Read the model definition and answer for the solid it produces. Units are mm, in the model's axes. Coordinates: 2 decimals unless noted, no trailing zeros. Order: outer loops, then holes, each group sorted by start corner. A loop starts at its lowest first (then second) coordinate and runs counter-clockwise, first axis right, second up. Notation, with made-up numbers: (88, -37.75) -> (121, -37.75) arc R20 ccw to (121, -27.75) -> close; hole circle Ø9 at (16.5, 38.25). An arc over 180 degrees is marked (long way). Answer in a Markdown table with one row per item.
from build123d import *

# Parameters (mm, degrees)
BOSS_EXTRUDE1_DEPTH = 1.5875
CUT_EXTRUDE1_DEPTH  = 4.175


with BuildPart() as part:
    # Sketch1 → Boss-Extrude1 (new body, symmetric)
    with BuildSketch(Plane.XY):
        Polygon((76.2, 37.697541537), (76.2, 56.747541537), (79.375, 56.747541537), (79.375, 37.697541537), (92.075, 37.697541537), (92.075, 46.587541537), (95.25, 46.587541537), (95.25, 37.697541537), (136.525, 37.697541537), (136.525, 46.587541537), (139.7, 46.587541537), (139.7, 37.697541537), (152.4, 37.697541537), (152.4, 69.447541537), (0, 69.447541537), (-0.423998633, 69.491926731), (-3.587863461, 69.757603883), (-946.051908629, 122.953392794), (-946.583462345, 116.623288424), (-943.412318182, 116.444298555), (-943.91275138, 110.48479854), (-6.775989292, 31.791225946), (-5.713280681, 44.446685258), (-2.549415853, 44.181008106), (-3.612124464, 31.525548794), (-1.492292584, 31.347541537), (0, 31.347541537), (0, 44.047541537), (3.175, 44.047541537), (3.175, 31.347541537), (15.875, 31.347541537), (15.875, 36.427541537), (19.05, 36.427541537), (19.05, 31.347541537), (25.4, 31.347541537), (69.85, 37.697541537), align=None)
    extrude(amount=BOSS_EXTRUDE1_DEPTH, both=True)

    # Sketch2 → Cut-Extrude1 (cut, through all)
    with BuildSketch(Plane.XY.offset(1.5875)):
        Polygon((-76.254460917, 37.625496217), (-75.245037036, 49.646404609), (-78.411328309, 49.883186), (-79.418325745, 37.891173369), align=None)
        Polygon((-155.224527027, 44.256797945), (-154.27566721, 55.556468134), (-157.441958483, 55.793249525), (-158.388391855, 44.522475098), align=None)
        Polygon((-234.194593137, 50.888099674), (-233.306297384, 61.466531659), (-236.472588657, 61.70331305), (-237.358457965, 51.153776826), align=None)
        Polygon((-313.164659247, 57.519401402), (-312.336927558, 67.376595183), (-315.503218831, 67.613376574), (-316.328524075, 57.785078555), align=None)
        Polygon((-392.134725356, 64.15070313), (-391.367557732, 73.286658708), (-394.533849005, 73.523440099), (-395.298590185, 64.416380283), align=None)
        Polygon((-471.104791466, 70.782004859), (-470.398187906, 79.196722233), (-473.564479179, 79.433503624), (-474.268656294, 71.047682011), align=None)
        Polygon((-550.074857576, 77.413306587), (-549.42881808, 85.106785757), (-552.595109353, 85.343567149), (-553.238722404, 77.67898374), align=None)
        Polygon((-629.044923686, 84.044608316), (-628.459448254, 91.016849282), (-631.625739527, 91.253630673), (-632.208788514, 84.310285468), align=None)
        Polygon((-708.014989796, 90.675910044), (-707.490078428, 96.926912807), (-710.656369701, 97.163694198), (-711.178854624, 90.941587197), align=None)
        Polygon((-786.985055905, 97.307211772), (-786.520708602, 102.836976331), (-789.686999875, 103.073757723), (-790.148920734, 97.572888925), align=None)
        Polygon((-865.955122015, 103.938513501), (-865.551338776, 108.747039856), (-868.717630049, 108.983821247), (-869.118986843, 104.204190653), align=None)
    extrude(amount=-CUT_EXTRUDE1_DEPTH, mode=Mode.SUBTRACT)


solid = part.part
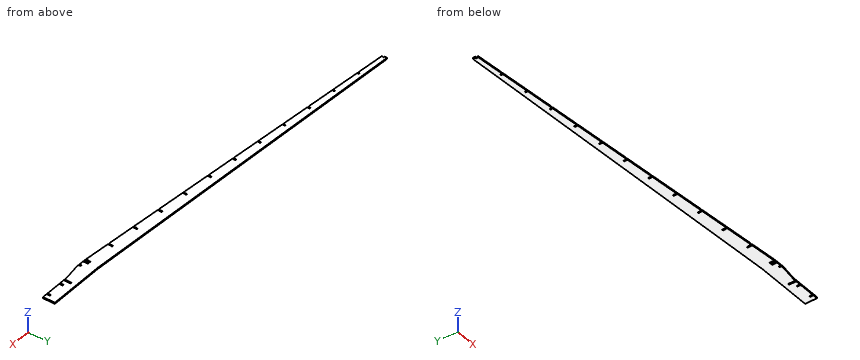
Q1. The part is cut by section B-B (x = -661). Write down the section's boundary in (y, z), then the cut area to 3 significant figures.
Outcome:
| item | result |
|---|---|
| outline | (86.73, -1.59) -> (106.86, -1.59) -> (106.86, 1.59) -> (86.73, 1.59) -> close |
| area | 63.9 mm² |
Q2. Given pin 1 (1 mm diameter, centred on x = 106.5, z = -0.5, fed in from -Y); pin 2 (1 mm diameter, centred on x = 94.5, z = 0, fed in from -Y); pin 3 (1.5 mm diameter, centred on x = -673.5, z = -1, fed in from -Y), each flat-ended and moving along its own axis, determine where each tip first touches the part or whether it passes through.
Outcome:
| item | result |
|---|---|
| pin 1 | y = 37.7 |
| pin 2 | y = 46.59 |
| pin 3 | y = 87.71 |
Q3. Consider line 1 (Y direction, x = -887.5, z = 1); line 2 (Y direction, x = 101.5, z = 0.95). Determine where each line is inside the solid, lowest interval first.
Outcome:
| item | result |
|---|---|
| line 1 | 105.75 to 119.65 |
| line 2 | 37.7 to 69.45 |
Q4. The part is cut by section A-A (x = -28). Write down the section's boundary in (y, z), then the cut area to 3 significant figures.
Outcome:
| item | result |
|---|---|
| outline | (33.57, -1.59) -> (71.14, -1.59) -> (71.14, 1.59) -> (33.57, 1.59) -> close |
| area | 119 mm² |
